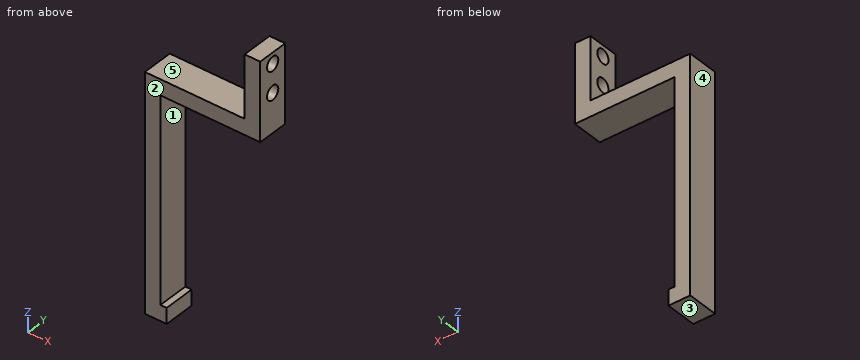
from build123d import *

# Parameters (mm, degrees)
BOSS_EXTRUDE1_DEPTH = 10
SKETCH3_R           = 2.25
CUT_EXTRUDE1_DEPTH  = 38


with BuildPart() as part:
    # Sketch2 → Boss-Extrude1 (new body)
    with BuildSketch(Plane(origin=(0, 0, 0), x_dir=(1, 0, 0), z_dir=(0, 1, 0))):
        Polygon((-5, 0), (0, 0), (0, 25), (-32, 25), (-32, 90), (-30, 90), (-30, 95), (-37, 95), (-37, 20), (-5, 20), align=None)
    extrude(amount=BOSS_EXTRUDE1_DEPTH)

    # Sketch3 → Cut-Extrude1 (cut, through all)
    with BuildSketch(Plane(origin=(0, 0, 0), x_dir=(0, 0, -1), z_dir=(1, 0, 0))):
        with Locations((3.5, 5)):
            Circle(SKETCH3_R)
        with Locations((12.5, 5)):
            Circle(SKETCH3_R)
    extrude(amount=-CUT_EXTRUDE1_DEPTH, mode=Mode.SUBTRACT)


solid = part.part
Geometry check sheet. Reference: the model listing, model coordinates, mm. Face numbers are marked on the shaded views. A direction names the side the tool comes from. Give positions to 0.01 mm unless a question says otherwise; leave off trailing zeros. Order: outer loops, then holes, each group sorted by start corner. A loop starts at its lowest first (then second) coordinate and runs counter-clockwise, first axis right, second up.
1) Cross-section at A-A (y = 5). Record the boundary of the cut face in (x, z).
Results are:
outline: (-37, -95) - (-30, -95) - (-30, -90) - (-32, -90) - (-32, -25) - (0, -25) - (0, -14.75) - (-5, -14.75) - (-5, -20) - (-37, -20) - close; (-5, -10.25) - (0, -10.25) - (0, -5.75) - (-5, -5.75) - close; (-5, -1.25) - (0, -1.25) - (0, 0) - (-5, 0) - close
2) Material ranges on probe 1 along Y at (x, z) = (-2.25, -12.5); probe 2 along Z at (x, y) = (-2, 3.5); probe 3 along X at (y, z) = (7, -87.5), recorded low to high.
Results are:
probe 1: y = 0 to 2.75, 7.25 to 10
probe 2: z = -25 to -14.18, -10.82 to -5.18, -1.82 to 0
probe 3: x = -37 to -32
3) Tool access check on the marked faces 4 and 5. Record the directions out of +Z, -Z, +X, -X, +Y, -Y that give a thin tool (end or side, any length) a straight path to the whole face; none if there is none.
Results are:
face 4: +Z, -Z, -X, +Y, -Y
face 5: +Z, -X, +Y, -Y
4) Cross-section at B-B (z = -12.5). Record the boundary of the cut face in (x, y).
Results are:
outline: (-5, 0) - (0, 0) - (0, 2.75) - (-5, 2.75) - close; (-5, 7.25) - (0, 7.25) - (0, 10) - (-5, 10) - close
5) Cross-section at C-C (x = -17). Record the boundary of the cut face in (y, z).
Results are:
outline: (0, -25) - (10, -25) - (10, -20) - (0, -20) - close
6) Gauge pin test, flat ends, axial feed: pin 1 (3 mm diameter, centred on x = -22.5, y = 5, fed in from -Z); pin 2 (3.5 mm diameter, centred on y = 5, z = -12.5, fed in from -X); pin 3 (4 mm diameter, centred on y = 2.5, z = -91.5, fed in from +X); pin 4 (6 mm diameter, centred on y = 2, z = -53, fed in from +X). Record the tip position at first contact, or that the pin passes through.
Results are:
pin 1: stops at z = -25
pin 2: passes through
pin 3: stops at x = -30
pin 4: stops at x = -32
7) Draft check along Z on the marked faces 1, 2 and 3. Enter one of: released by +Z, released by -Z, zero draft, split by the parting line, or undercut.
Results are:
face 1: undercut
face 2: zero draft
face 3: released by -Z
8) Cross-section at D-D (z = -44). Record the boundary of the cut face in (x, y), then the cut area to 3 significant figures.
Results are:
outline: (-37, 0) - (-32, 0) - (-32, 10) - (-37, 10) - close
area: 50.0 mm2
